```python
from build123d import *

# Parameters (mm, degrees)
BOSS_EXTRUDE1_DEPTH = 35.5
BOSS_EXTRUDE2_START = 5
SKETCH2_W           = 90
SKETCH2_H           = 80
SKETCH2_R           = 2
BOSS_EXTRUDE2_DEPTH = 5
BOSS_EXTRUDE3_DEPTH = 3
SKETCH4_R           = 1.5
CUT_EXTRUDE1_DEPTH  = 3
SKETCH5_W           = 4
SKETCH5_H           = 4
CUT_EXTRUDE2_DEPTH  = 72.465026412


with BuildPart() as part:
    # Sketch1 → Boss-Extrude1 (new body)
    with BuildSketch(Plane.XY):
        with BuildLine():
            Line((-23, 0), (-19, 0))
            ThreePointArc((-19, 0), (0, -19), (19, 0))
            Line((19, 0), (23, 0))
            ThreePointArc((23, 0), (0, -23), (-23, 0))
        make_face()
    extrude(amount=BOSS_EXTRUDE1_DEPTH)

    # Sketch2 → Boss-Extrude2 (add)
    # profile 1 of 2: a face of its own
    with BuildSketch(Plane(origin=(0, 0, 0), x_dir=(-1, 0, 0), z_dir=(0, 0, -1)).offset(BOSS_EXTRUDE2_START)):
        Rectangle(SKETCH2_W, SKETCH2_H)
        with Locations((39.020725451, 34.685089289)):
            Circle(SKETCH2_R, mode=Mode.SUBTRACT)
        with Locations((-39.020725451, 34.685089289)):
            Circle(SKETCH2_R, mode=Mode.SUBTRACT)
        with Locations((39.020725451, -34.685089289)):
            Circle(SKETCH2_R, mode=Mode.SUBTRACT)
        with Locations((-39.020725451, -34.685089289)):
            Circle(SKETCH2_R, mode=Mode.SUBTRACT)
        with BuildLine():
            Line((23, 0), (19, 0))
            ThreePointArc((19, 0), (0, -19), (-19, 0))
            Line((-19, 0), (-23, 0))
            ThreePointArc((-23, 0), (0, -23), (23, 0))
        make_face(mode=Mode.SUBTRACT)
    # profile 2 of 2: a face of its own
    with BuildSketch(Plane(origin=(0, 0, 0), x_dir=(-1, 0, 0), z_dir=(0, 0, -1)).offset(BOSS_EXTRUDE2_START)):
        with BuildLine():
            ThreePointArc((-23, 0), (0, -23), (23, 0))
            Line((23, 0), (19, 0))
            ThreePointArc((19, 0), (0, -19), (-19, 0))
            Line((-19, 0), (-23, 0))
        make_face()
    extrude(amount=-BOSS_EXTRUDE2_DEPTH)

    # Sketch3 → Boss-Extrude3 (add)
    with BuildSketch(Plane.XY.offset(35.5)):
        with BuildLine():
            Line((-23, 0), (-10, 0))
            ThreePointArc((-10, 0), (0, -10), (10, 0))
            Line((10, 0), (23, 0))
            ThreePointArc((23, 0), (0, -23), (-23, 0))
        make_face()
    extrude(amount=BOSS_EXTRUDE3_DEPTH)

    # Sketch4 → Cut-Extrude1 (cut)
    with BuildSketch(Plane.XY.offset(38.5)):
        with Locations((-9.536891354, -10.249278184)):
            Circle(SKETCH4_R)
        with Locations((13.644580955, -3.134551093)):
            Circle(SKETCH4_R)
        with Locations((10.049016147, -11.136304346)):
            Circle(SKETCH4_R)
        with Locations((-14.668830541, -3.134551093)):
            Circle(SKETCH4_R)
    extrude(amount=-CUT_EXTRUDE1_DEPTH, mode=Mode.SUBTRACT)

    # Sketch5 → Cut-Extrude2 (cut, through all)
    with BuildSketch(Plane.XY):
        with Locations((-12, 24)):
            Rectangle(SKETCH5_W, SKETCH5_H)
        with Locations((-2, 24)):
            Rectangle(SKETCH5_W, SKETCH5_H)
    extrude(amount=-CUT_EXTRUDE2_DEPTH, mode=Mode.SUBTRACT)


solid = part.part
```
Work out the finished part from the listing and answer in its coordinate system (mm). A direction names the side the tool comes from. Round coordinates to 2 decimals unless told otherwise and drop trailing zeros. Order: outer loops, then holes, each group sorted by start corner. A loop starts at its lowest first (then second) coordinate and runs counter-clockwise, first axis right, second up.
Q1. The mould has two halves that part along Z. Classify faces 4 (the flat face through (1, -40, -3)), 5 (the flat face through (1, 1, -5)), 6 (the cylindrical face through (0, -19, 18)): pulls with the +Z half, pulls with the -Z half, needs draft (parallel to the pull), parting line crosses it, or undercut.
Solution:
face 4: needs draft
face 5: pulls with the -Z half
face 6: undercut
Q2. Given pin 1 Ø1.8 at (x, y) = (10.05, -11.14) entering from +Z; pin 2 Ø5 at (x, z) = (2.5, 33.5) entering from +Y; pin 3 Ø5 at (y, z) = (-13.5, 19.5) entering from +X; pin 4 Ø4 at (x, y) = (13.64, -3.13) entering from +Z, each flat-ended and moving along its own axis, determine where each tip first touches the part or whether it passes through.
Solution:
pin 1: stops at z = 0
pin 2: stops at y = -9.17
pin 3: stops at x = 20.2
pin 4: stops at z = 38.5
Q3. A tool of negligible diameter and unlimited length cuts with its end or side. For faces 1 (the cylindrical face through (-13.283, -3.709, 37.021)), 2 (the flat face through (-14, 24, -2)), 3 (the cylindrical face through (0.506, -22.994, 18.98)), from which of +Z, -Z, +X, -X, +Y, -Y can it reach the whole face along a straight path? Write none if from no direction.
Solution:
face 1: +Z
face 2: +Z, -Z
face 3: +Z, -Y
Q4. Find the intervals of material crossed by line 1 along Z through (x, y) = (-23, 18); line 2 along Y through (x, z) = (-3, -3); line 3 along X through (y, z) = (-4.5, 37.5), in increasing order.
Solution:
line 1: z = -5 to 0
line 2: y = -40 to 22, 26 to 40
line 3: x = -22.56 to -15.29, -14.05 to -8.93, 8.93 to 13.02, 14.27 to 22.56
Q5. A cutting plane is placed at A-A, the plane y = 20. Determine the outline of the cut face in (x, z).
Solution:
outline: (-45, -5) - (45, -5) - (45, 0) - (-45, 0) - close
Q6. A cutting plane is placed at B-B, the plane z = 16.5. Determine the outline of the cut face in (x, y).
Solution:
outline: (-23, 0) arc R23 ccw to (23, 0) - (19, 0) arc R19 cw to (-19, 0) - close
